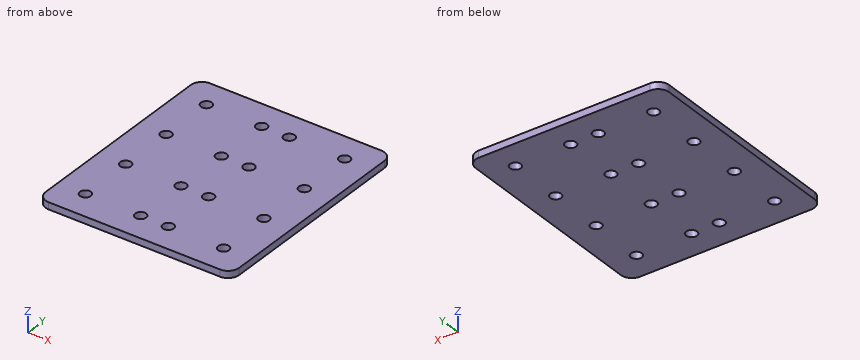
from build123d import *

# Parameters (mm, degrees)
SKETCH1_R           = 2.5
BOSS_EXTRUDE1_DEPTH = 3.175


with BuildPart() as part:
    # Sketch1 → Boss-Extrude1 (new body)
    with BuildSketch(Plane.XY):
        with BuildLine():
            Line((1176.02, 25.4), (1097.28, 25.4))
            ThreePointArc((1097.28, 25.4), (1093.687897552, 23.912102448), (1092.2, 20.32))
            Line((1092.2, 20.32), (1092.2, -71.12))
            ThreePointArc((1092.2, -71.12), (1093.687897552, -74.712102448), (1097.28, -76.2))
            Line((1097.28, -76.2), (1176.02, -76.2))
            ThreePointArc((1176.02, -76.2), (1179.612102448, -74.712102448), (1181.1, -71.12))
            Line((1181.1, -71.12), (1181.1, 20.32))
            ThreePointArc((1181.1, 20.32), (1179.612102448, 23.912102448), (1176.02, 25.4))
        make_face()
        with Locations((1143, 12.7)):
            Circle(SKETCH1_R, mode=Mode.SUBTRACT)
        with Locations((1168.4, 12.7)):
            Circle(SKETCH1_R, mode=Mode.SUBTRACT)
        with Locations((1168.4, -12.7)):
            Circle(SKETCH1_R, mode=Mode.SUBTRACT)
        with Locations((1168.4, -38.1)):
            Circle(SKETCH1_R, mode=Mode.SUBTRACT)
        with Locations((1168.4, -63.5)):
            Circle(SKETCH1_R, mode=Mode.SUBTRACT)
        with Locations((1143, -12.7)):
            Circle(SKETCH1_R, mode=Mode.SUBTRACT)
        with Locations((1143, -38.1)):
            Circle(SKETCH1_R, mode=Mode.SUBTRACT)
        with Locations((1143, -63.5)):
            Circle(SKETCH1_R, mode=Mode.SUBTRACT)
        with Locations(Location((1104.9, 12.7, 0), (0, 0, 180))):
            Circle(SKETCH1_R, mode=Mode.SUBTRACT)
        with Locations(Location((1104.9, -12.7, 0), (0, 0, 180))):
            Circle(SKETCH1_R, mode=Mode.SUBTRACT)
        with Locations(Location((1104.9, -38.1, 0), (0, 0, 180))):
            Circle(SKETCH1_R, mode=Mode.SUBTRACT)
        with Locations(Location((1104.9, -63.5, 0), (0, 0, 180))):
            Circle(SKETCH1_R, mode=Mode.SUBTRACT)
        with Locations(Location((1130.3, -63.5, 0), (0, 0, 180))):
            Circle(SKETCH1_R, mode=Mode.SUBTRACT)
        with Locations(Location((1130.3, -38.1, 0), (0, 0, 180))):
            Circle(SKETCH1_R, mode=Mode.SUBTRACT)
        with Locations(Location((1130.3, -12.7, 0), (0, 0, 180))):
            Circle(SKETCH1_R, mode=Mode.SUBTRACT)
        with Locations(Location((1130.3, 12.7, 0), (0, 0, 180))):
            Circle(SKETCH1_R, mode=Mode.SUBTRACT)
    extrude(amount=BOSS_EXTRUDE1_DEPTH)


solid = part.part
Could you check a few things on this model? Use its own coordinates, in mm. Round coordinates to 2 decimals unless told otherwise and drop trailing zeros. Loops run counter-clockwise (first coordinate to the right, second up) from the corner with the lowest first, then second, coordinate; pieces in that order, holes last. Notation, with made-up numbers: (38.25, -7.75) - (75.25, -7.75) arc R28 cw to (75.25, 20.25) - close; hole circle Ø11 at (-10, 29.25). An arc over 180 degrees is marked (long way). Write item = value, one per line.
1) Imagine slicing it at A-A (x = 1104.9). Please give me the cut outline in (y, z) (3 decimals).
Computed:
outline = (-76.2, 0) - (-66, 0) - (-66, 3.175) - (-76.2, 3.175) - close; (-61, 0) - (-40.6, 0) - (-40.6, 3.175) - (-61, 3.175) - close; (-35.6, 0) - (-15.2, 0) - (-15.2, 3.175) - (-35.6, 3.175) - close; (-10.2, 0) - (10.2, 0) - (10.2, 3.175) - (-10.2, 3.175) - close; (15.2, 0) - (25.4, 0) - (25.4, 3.175) - (15.2, 3.175) - close
2) Imagine slicing it at C-C (z = 1.5). Give the number of separate pieces and of enclosed holes in the cut face, and give its area (3 significant figures).
Computed:
separate_pieces = 1
enclosed_holes = 16
area = 8,700 mm2
3) I need wall thicknesses on line 1 along Y through (x, z) = (1104.9, 2.1); line 2 along X through (y, z) = (-62, 0.2); line 3 along X through (y, z) = (-71.5, 0.4). Which ranges of each line are inside material? Lowest first, please. Write a range as from..to.
Computed:
line_1 = -76.2..-66, -61..-40.6, -35.6..-15.2, -10.2..10.2, 15.2..25.4
line_2 = 1092.2..1102.9, 1106.9..1128.3, 1132.3..1141, 1145..1166.4, 1170.4..1181.1
line_3 = 1092.21..1181.09
4) I'm going to push a flat-ended pin straight in: P1, Ø4, axis at x = 1143, y = -12.7, coming from the +Z side. Where does the tip first touch, or does it pass through?
Computed:
P1 = through
5) Imagine slicing it at B-B (y = -63.5). Please give me the cut outline in (x, z) (3 decimals), and give its area (3 significant figures).
Computed:
outline = (1092.2, 0) - (1102.4, 0) - (1102.4, 3.175) - (1092.2, 3.175) - close; (1107.4, 0) - (1127.8, 0) - (1127.8, 3.175) - (1107.4, 3.175) - close; (1132.8, 0) - (1140.5, 0) - (1140.5, 3.175) - (1132.8, 3.175) - close; (1145.5, 0) - (1165.9, 0) - (1165.9, 3.175) - (1145.5, 3.175) - close; (1170.9, 0) - (1181.1, 0) - (1181.1, 3.175) - (1170.9, 3.175) - close
area = 219 mm2
